Check sheet for the modelled part. Datum: model origin and axes. Units: mm. A direction names the side the tool comes from. Give positions to 0.01 mm unless a question says otherwise; leave off trailing zeros. Loops run counter-clockwise (first coordinate to the right, second up) from the corner with the lowest first, then second, coordinate; pieces in that order, holes last. Notation, with made-up numbers: (31, 26.5) - (70, 26.5) arc R20 ccw to (70, 44.5) - close; hole circle Ø9 at (77.5, 49). An arc over 180 degrees is marked (long way). Use CSV: the item, a comma, the result in double quotes.
from build123d import *

# Parameters (mm, degrees)
F0_R     = 63.5
F1_DEPTH = 36.83
F2_R     = 50.8
F3_DEPTH = 25.4
F4_W     = 38.1
F4_H     = 38.1
F5_DEPTH = 25.4


with BuildPart() as f1:
    # F0 (on Front) → F1 (new body)
    with BuildSketch(Plane.XZ):
        Circle(F0_R)
    extrude(amount=F1_DEPTH)

    # F2 (on face) → F3 (cut)
    with BuildSketch(Plane.XZ.offset(36.83)):
        Circle(F2_R)
    extrude(amount=-F3_DEPTH, mode=Mode.SUBTRACT)

    # F4 (on face) → F5 (cut)
    with BuildSketch(Plane(origin=(0, 0, 0), x_dir=(-1, 0, 0), z_dir=(0, 1, 0))):
        Rectangle(F4_W, F4_H)
    extrude(amount=-F5_DEPTH, mode=Mode.SUBTRACT)


solid = f1.part
1. Set-up check for faces 4 (the face through (27, 0, 1)), 5 (the face through (-11.012, -24.308, -49.592)), 6 (the face through (-19.05, -6, 0)): record each of +Z, -Z, +X, -X, +Y, -Y from which the full face is reachable in a straight line by a thin tool's end or side.
Completed:
face 4,"+Z, -Z, +X, -X, +Y"
face 5,"-Y"
face 6,"+Y, -Y"
2. Sectioned sample at B-B, the plane x = 0. Record the boundary of the cut face in (y, z), and give its area (3 significant figures).
Completed:
outline,"(-36.83, -63.5) - (0, -63.5) - (0, -19.05) - (-11.43, -19.05) - (-11.43, -50.8) - (-36.83, -50.8) - close; (-36.83, 50.8) - (-11.43, 50.8) - (-11.43, 19.05) - (0, 19.05) - (0, 63.5) - (-36.83, 63.5) - close"
area,"1,660 mm²"
3. Release check for a two-part mould opening along Z. For faces 1 (the face through (-13.77, -18.16, -61.99)), 2 (the face through (-29, -36.83, 43)), 3 (the face through (0, -6, -19.05)) record: released by +Z, released by -Z, zero draft, split by the parting line, or undercut.
Completed:
face 1,"split by the parting line"
face 2,"zero draft"
face 3,"undercut"
4. Sectioned sample at D-D, the plane z = 45. Record the boundary of the cut face in (x, y), and give its area (3 significant figures).
Completed:
outline,"(-44.8, -36.83) - (-23.57, -36.83) - (-23.57, -11.43) - (23.57, -11.43) - (23.57, -36.83) - (44.8, -36.83) - (44.8, 0) - (-44.8, 0) - close"
area,"2,100 mm²"
5. Go/stop test with flat-tipped pins: pin 1 Ø12.5 at (x, y) = (4, -4) entering from +Z; pin 2 Ø5 at (x, z) = (-24, 9) entering from -Y; pin 3 Ø6 at (y, z) = (-15, -23) entering from +X. Record where each tip stops, or that it passes through.
Completed:
pin 1,"stops at z = 63.5"
pin 2,"stops at y = -11.43"
pin 3,"stops at x = 60.27"
6. Scan lines: line 1 along Z through (x, y) = (0, -20.25); line 2 along X through (y, z) = (-11.5, 21); line 3 along X through (y, z) = (-31, -42). Record each from-to range of solid material in increasing order.
Completed:
line 1,"z = -63.5 to -50.8, 50.8 to 63.5"
line 2,"x = -59.93 to -46.26, 46.26 to 59.93"
line 3,"x = -47.63 to -28.58, 28.58 to 47.63"
7. Sectioned sample at A-A, the plane z = 0. Record the boundary of the cut face in (x, y).
Completed:
outline,"(-63.5, -36.83) - (-50.8, -36.83) - (-50.8, -11.43) - (-19.05, -11.43) - (-19.05, 0) - (-63.5, 0) - close; (19.05, -11.43) - (50.8, -11.43) - (50.8, -36.83) - (63.5, -36.83) - (63.5, 0) - (19.05, 0) - close"
8. Sectioned sample at C-C, the plane y = -31. Record the boundary of the cut face in (x, z), and give its area (3 significant figures).
Completed:
outline,"circle Ø127 at (0, 0); hole circle Ø101.6 at (0, 0)"
area,"4,560 mm²"
